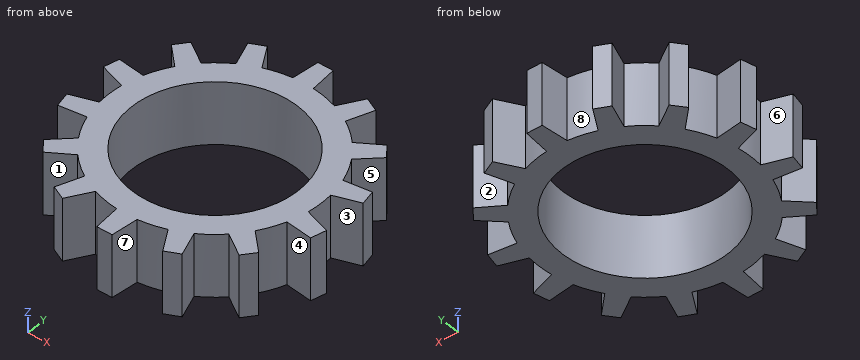
from build123d import *

# Parameters (mm, degrees)
CROQUIS1_R              = 4
SALIENTE_EXTRUIR1_DEPTH = 3


with BuildPart() as part:
    # Croquis1 → Saliente-Extruir1 (new body)
    with BuildSketch(Plane.XY):
        with BuildLine():
            Line((-0.5, 5.111716619), (-0.375, 6.411716619))
            Line((-0.375, 6.411716619), (0.375, 6.411716619))
            Line((0.375, 6.411716619), (0.5, 5.111716619))
            ThreePointArc((0.5, 5.111716619), (1.142892446, 5.007338979), (1.767406286, 4.822439404))
            Line((1.767406286, 4.822439404), (2.444076255, 5.939463465))
            Line((2.444076255, 5.939463465), (3.119802906, 5.614050661))
            Line((3.119802906, 5.614050661), (2.668375154, 4.388555665))
            ThreePointArc((2.668375154, 4.388555665), (3.202313472, 4.015574083), (3.684756081, 3.578018923))
            Line((3.684756081, 3.578018923), (4.779073233, 4.29082673))
            Line((4.779073233, 4.29082673), (5.246690585, 3.704453118))
            Line((5.246690585, 3.704453118), (4.308245883, 2.79618744))
            ThreePointArc((4.308245883, 2.79618744), (4.627477041, 2.228475492), (4.872294744, 1.624927912))
            Line((4.872294744, 1.624927912), (6.167516146, 1.792339137))
            Line((6.167516146, 1.792339137), (6.334406847, 1.061143203))
            Line((6.334406847, 1.061143203), (5.094815678, 0.65))
            ThreePointArc((5.094815678, 0.65), (5.13611203, 0), (5.094815678, -0.65))
            Line((5.094815678, -0.65), (6.334406847, -1.061143203))
            Line((6.334406847, -1.061143203), (6.167516146, -1.792339137))
            Line((6.167516146, -1.792339137), (4.872294744, -1.624927912))
            ThreePointArc((4.872294744, -1.624927912), (4.627477041, -2.228475492), (4.308245883, -2.79618744))
            Line((4.308245883, -2.79618744), (5.246690585, -3.704453118))
            Line((5.246690585, -3.704453118), (4.779073233, -4.29082673))
            Line((4.779073233, -4.29082673), (3.684756081, -3.578018923))
            ThreePointArc((3.684756081, -3.578018923), (3.202313472, -4.015574083), (2.668375154, -4.388555665))
            Line((2.668375154, -4.388555665), (3.119802906, -5.614050661))
            Line((3.119802906, -5.614050661), (2.444076255, -5.939463465))
            Line((2.444076255, -5.939463465), (1.767406286, -4.822439404))
            ThreePointArc((1.767406286, -4.822439404), (1.142892446, -5.007338979), (0.5, -5.111716619))
            Line((0.5, -5.111716619), (0.375, -6.411716619))
            Line((0.375, -6.411716619), (-0.375, -6.411716619))
            Line((-0.375, -6.411716619), (-0.5, -5.111716619))
            ThreePointArc((-0.5, -5.111716619), (-1.142892446, -5.007338979), (-1.767406286, -4.822439404))
            Line((-1.767406286, -4.822439404), (-2.444076255, -5.939463465))
            Line((-2.444076255, -5.939463465), (-3.119802906, -5.614050661))
            Line((-3.119802906, -5.614050661), (-2.668375154, -4.388555665))
            ThreePointArc((-2.668375154, -4.388555665), (-3.202313472, -4.015574083), (-3.684756081, -3.578018923))
            Line((-3.684756081, -3.578018923), (-4.779073233, -4.29082673))
            Line((-4.779073233, -4.29082673), (-5.246690585, -3.704453118))
            Line((-5.246690585, -3.704453118), (-4.308245883, -2.79618744))
            ThreePointArc((-4.308245883, -2.79618744), (-4.627477041, -2.228475492), (-4.872294744, -1.624927912))
            Line((-4.872294744, -1.624927912), (-6.167516146, -1.792339137))
            Line((-6.167516146, -1.792339137), (-6.334406847, -1.061143203))
            Line((-6.334406847, -1.061143203), (-5.094815678, -0.65))
            ThreePointArc((-5.094815678, -0.65), (-5.13611203, 0), (-5.094815678, 0.65))
            Line((-5.094815678, 0.65), (-6.334406847, 1.061143203))
            Line((-6.334406847, 1.061143203), (-6.167516146, 1.792339137))
            Line((-6.167516146, 1.792339137), (-4.872294744, 1.624927912))
            ThreePointArc((-4.872294744, 1.624927912), (-4.627477041, 2.228475492), (-4.308245883, 2.79618744))
            Line((-4.308245883, 2.79618744), (-5.246690585, 3.704453118))
            Line((-5.246690585, 3.704453118), (-4.779073233, 4.29082673))
            Line((-4.779073233, 4.29082673), (-3.684756081, 3.578018923))
            ThreePointArc((-3.684756081, 3.578018923), (-3.202313472, 4.015574083), (-2.668375154, 4.388555665))
            Line((-2.668375154, 4.388555665), (-3.119802906, 5.614050661))
            Line((-3.119802906, 5.614050661), (-2.444076255, 5.939463465))
            Line((-2.444076255, 5.939463465), (-1.767406286, 4.822439404))
            ThreePointArc((-1.767406286, 4.822439404), (-1.142892446, 5.007338979), (-0.5, 5.111716619))
        make_face()
        Circle(CROQUIS1_R, mode=Mode.SUBTRACT)
    extrude(amount=SALIENTE_EXTRUIR1_DEPTH)


solid = part.part
Work out the finished part from the listing and answer in its coordinate system (mm). Face numbers are marked on the shaded views. A direction names the side the tool comes from. Coordinates: 2 decimals unless noted, no trailing zeros. Loops run counter-clockwise (first coordinate to the right, second up) from the corner with the lowest first, then second, coordinate; pieces in that order, holes last. Notation, with made-up numbers: M 21,33 L 55,33 A17 ccw 55,52 Z; hole C -12.5,13.25 d3. An arc over 180 degrees is marked long. Answer in a Markdown table with one row per item. Add a question column.
1. A tool of negligible diameter and unlimited length cuts with its end or side. For the marked faces 5, 6, 7 and 8, from which of +Z, -Z, +X, -X, +Y, -Y can it reach the whole face along a straight path? Write none if from no direction.
2. Find section A-A, the plane y = 0. Write down the section's boundary in (x, z).
3. Find section B-B, the plane x = 0. Write down the section's boundary in (y, z).
4. A flat-ended cylindrical pin translates along its axis: P1, Ø1, axis at y = 4.5, z = 1, coming from the -X side. Find the tip coordinate at first contact, or state that the pin passes through.
5. Consider L1, parallel to Y at x = 0, z = 1.4; L2, parallel to X at y = -5.5, z = 0.4; L3, parallel to Y at x = -2.25, z = 2.5. Determine where each line is inside the solid, lowest interval first.
6. The mould has two halves that part along Y. Classify the marked faces 1, 2, 3 and 4: pulls with the +Y half, pulls with the -Y half, needs draft (parallel to the pull), parting line crosses it, or undercut.
Reported:
| question | item | result |
|---|---|---|
| 1 | face 5 | +Z, -Z, +X |
| 1 | face 6 | +Z, -Z, -X |
| 1 | face 7 | +Z, -Z, -Y |
| 1 | face 8 | +Z, -Z, +Y |
| 2 | outline | M -5.14,0 L -4,0 L -4,3 L -5.14,3 Z; M 4,0 L 5.14,0 L 5.14,3 L 4,3 Z |
| 3 | outline | M -6.41,0 L -4,0 L -4,3 L -6.41,3 Z; M 4,0 L 6.41,0 L 6.41,3 L 4,3 Z |
| 4 | P1 | stops at x = -5.01 |
| 5 | L1 | y = -6.41 to -4, 4 to 6.41 |
| 5 | L2 | x = -3.08 to -2.18, -0.46 to 0.46, 2.18 to 3.08 |
| 5 | L3 | y = -5.62 to -3.31, 3.31 to 5.62 |
| 6 | face 1 | pulls with the -Y half |
| 6 | face 2 | pulls with the +Y half |
| 6 | face 3 | undercut |
| 6 | face 4 | undercut |
